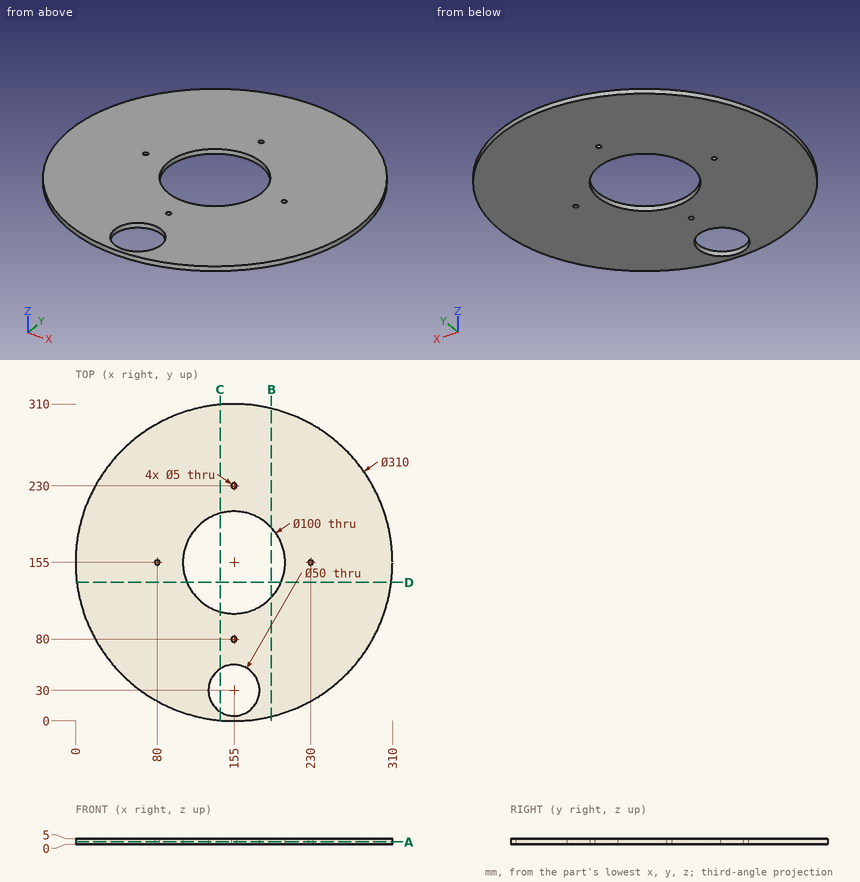
Source: three-view drawing plus pictorial views. Frame: mm from the lowest corner of the part. Round coordinates to 2 decimals unless told otherwise and drop trailing zeros. Loops run counter-clockwise (first coordinate to the right, second up) from the corner with the lowest first, then second, coordinate; pieces in that order, holes last.
Q1. Section D-D, the plane y = 135.5. Return loops of the section in (x, z).
Q2. Section A-A, the plane z = 2.2. Return loops of the section in (x, y), plus the area to 3 significant figures.
Q3. Ray query, line 1 (Y direction, x = 155, z = 3.1); line 2 (Y direction, x = 164, z = 0.6); line 3 (Y direction, x = 149.5, z = 1.6). Return the intervals inside material, ascending.
Q4. Section C-C, the plane x = 141.5. Return loops of the section in (y, z), plus the area to 3 significant figures.
Q5. Section B-B, the plane x = 191.5. Return loops of the section in (y, z).
Q6. First-contact query: P1, Ø3, axis at x = 155, y = 230, coming from the +Z side; P2, Ø1.5, axis at y = 91, z = 2.5, coming from the -X side; P3, Ø1.5, axis at x = 57, z = 1, coming from the -Y side. Flat tips, straight axial feed; report the tip coordinate or a pass-through.
Solutions:
1. outline: (1.23, 0) - (108.96, 0) - (108.96, 5) - (1.23, 5) - close; (201.04, 0) - (308.77, 0) - (308.77, 5) - (201.04, 5) - close
2. outline: circle Ø310 at (155, 155); hole circle Ø5 at (80, 155); hole circle Ø100 at (155, 155); hole circle Ø50 at (155, 30); hole circle Ø5 at (155, 80); hole circle Ø5 at (155, 230); hole circle Ø5 at (230, 155)
2. area: 65,600 mm2
3. line 1: y = 0 to 5, 55 to 77.5, 82.5 to 105, 205 to 227.5, 232.5 to 310
3. line 2: y = 0.26 to 6.68, 53.32 to 105.82, 204.18 to 309.74
3. line 3: y = 0.1 to 5.61, 54.39 to 105.3, 204.7 to 309.9
4. outline: (0.59, 0) - (8.96, 0) - (8.96, 5) - (0.59, 5) - close; (51.04, 0) - (106.86, 0) - (106.86, 5) - (51.04, 5) - close; (203.14, 0) - (309.41, 0) - (309.41, 5) - (203.14, 5) - close
4. area: 852 mm2
5. outline: (4.36, 0) - (120.83, 0) - (120.83, 5) - (4.36, 5) - close; (189.17, 0) - (305.64, 0) - (305.64, 5) - (189.17, 5) - close
6. P1: passes through
6. P2: stops at x = 13.49
6. P3: stops at y = 34.3
